```python
from build123d import *

# Parameters (mm, degrees)
F0_R     = 2.55
F1_DEPTH = 6.1
F3_DEPTH = 2.5
F6_DEPTH = 1.2


with BuildPart() as f1:
    # F0 (on Top) → F1 (new body)
    with BuildSketch(Plane.XY):
        with BuildLine():
            ThreePointArc((-22.8091472875, 20.7166310371), (-24.4512119604, 22.7321355607), (-25.1048969271, 25.2483491523))
            ThreePointArc((-25.1048969271, 25.2483491523), (-34.1357153903, 30.6750208196), (-35.5153225806, 20.2298721131))
            ThreePointArc((-35.5153225806, 20.2298721131), (-33.9539864651, 18.15120321), (-33.4, 15.6111768576))
            Line((-33.4, 15.6111768576), (-33.4, -15.6111768576))
            ThreePointArc((-33.4, -15.6111768576), (-33.9539864651, -18.15120321), (-35.5153225806, -20.2298721131))
            ThreePointArc((-35.5153225806, -20.2298721131), (-34.1357149704, -30.6750210221), (-25.1048968903, -25.2483482207))
            ThreePointArc((-25.1048968903, -25.2483482207), (-24.4512125214, -22.7321357825), (-22.8091487233, -20.7166321802))
            Line((-22.8091487233, -20.7166321802), (-16.801235426, -15.9332617206))
            ThreePointArc((-16.801235426, -15.9332617206), (-16.4823258273, -13.1228708816), (-19.2927166663, -12.8039612829))
            Line((-19.2927166663, -12.8039612829), (-25.3006299635, -17.5873317424))
            ThreePointArc((-25.3006299635, -17.5873317424), (-27.9708920533, -17.8865901621), (-29.4, -15.6111768576))
            Line((-29.4, -15.6111768576), (-29.4, 15.6111768576))
            ThreePointArc((-29.4, 15.6111768576), (-27.9708912267, 17.8865905605), (-25.3006285278, 17.5873305993))
            Line((-25.3006285278, 17.5873305993), (-8.5908527125, 4.2833689629))
            ThreePointArc((-8.5908527125, 4.2833689629), (-6.5260006587, 0), (-8.5908527125, -4.2833689629))
            Line((-8.5908527125, -4.2833689629), (-14.5987660097, -9.0667394225))
            ThreePointArc((-14.5987660097, -9.0667394225), (-14.9176756084, -11.8771302615), (-12.1072847694, -12.1960398602))
            Line((-12.1072847694, -12.1960398602), (-6.0993714722, -7.4126694007))
            ThreePointArc((-6.0993714722, -7.4126694007), (-3.7671833568, -6.2639599209), (-1.1684785693, -6.1906912242))
            ThreePointArc((-1.1684785693, -6.1906912242), (6.3, 0), (-1.1684785693, 6.1906912242))
            ThreePointArc((-1.1684785693, 6.1906912242), (-3.7671833568, 6.2639599209), (-6.0993714722, 7.4126694007))
            Line((-6.0993714722, 7.4126694007), (-22.8091472875, 20.7166310371))
        make_face()
        with Locations((-31.4, -25)):
            Circle(F0_R, mode=Mode.SUBTRACT)
        with Locations((-31.4, 25)):
            Circle(F0_R, mode=Mode.SUBTRACT)
        Circle(F0_R, mode=Mode.SUBTRACT)
    extrude(amount=F1_DEPTH)

    # F2 (on face) → F3 (cut)
    with BuildSketch(Plane.XY.offset(6.1)):
        Polygon((-27.35, 22.6617314098), (-27.35, 27.3382685902), (-31.4, 29.6765371804), (-35.45, 27.3382685902), (-35.45, 22.6617314098), (-31.4, 20.3234628196), align=None)
        Polygon((-27.35, -27.3382685902), (-27.35, -22.6617314098), (-31.4, -20.3234628196), (-35.45, -22.6617314098), (-35.45, -27.3382685902), (-31.4, -29.6765371804), align=None)
        Polygon((-4.05, 2.3382685902), (-4.05, -2.3382685902), (0, -4.6765371804), (4.05, -2.3382685902), (4.05, 2.3382685902), (0, 4.6765371804), align=None)
    extrude(amount=-F3_DEPTH, mode=Mode.SUBTRACT)

    # F5 (on mid) → F6 (cut, symmetric)
    with BuildSketch(Plane.XY.offset(3.05)):
        with BuildLine():
            Line((-19.2927166663, -12.8039612829), (-21.5397744668, -14.5930200413))
            ThreePointArc((-21.5397744668, -14.5930200413), (-20.7851139292, -16.5486575869), (-19.0482932266, -17.722320479))
            Line((-19.0482932266, -17.722320479), (-16.801235426, -15.9332617206))
            ThreePointArc((-16.801235426, -15.9332617206), (-19.611626265, -15.6143521218), (-19.2927166663, -12.8039612829))
        make_face()
        with BuildLine():
            ThreePointArc((-14.5987660097, -9.0667394225), (-11.7883751707, -9.3856490213), (-12.1072847694, -12.1960398602))
            Line((-12.1072847694, -12.1960398602), (-9.8602269689, -10.4069811018))
            ThreePointArc((-9.8602269689, -10.4069811018), (-10.6148875066, -8.4513435562), (-12.3517082091, -7.2776806641))
            Line((-12.3517082091, -7.2776806641), (-14.5987660097, -9.0667394225))
        make_face()
    extrude(amount=F6_DEPTH, both=True, mode=Mode.SUBTRACT)


solid = f1.part
```
Can you work these out from the model? Positions are in its coordinate system, mm. A direction names the side the tool comes from. Coordinates: 2 decimals unless noted, no trailing zeros. Order: outer loops, then holes, each group sorted by start corner. A loop starts at its lowest first (then second) coordinate and runs counter-clockwise, first axis right, second up.
1. If we section it at C-C (y = -19): Please give me the cut outline in (x, z).
2. Thinking about a two-plate mould opening in X: for faces 6 (the face through (-33.969, 18.185, 3.007)), 7 (the face through (-24.468, -22.765, 3.007)), 8 (the face through (-30.03, 27.15, 1.77)), which applies, +X half, -X half, draft (parallel to the pull), parting line (faces both ways), or undercut?
3. I'm going to push flat-ended pins straight in: pin 1 (3 mm diameter, centred on y = 0, z = 4.5, fed in from -X); pin 2 (3 mm diameter, centred on x = -4, z = 4.5, fed in from -Y); pin 3 (1 mm diameter, centred on y = -18, z = 1.5, fed in from -X). Where does each tip first touch, or does it pass through?
4. If we section it at A-A (y = 0): Please give me the cut outline in (x, z).
5. If we section it at B-B (z = 2.75): Please give me the cut outline in (x, y).
6. I need wall thicknesses on line 1 (Y direction, x = -31.4, z = 1.9); line 2 (Y direction, x = 0, z = 1.95); line 3 (X direction, y = -3.5, z = 5). Which ranges of each line are inside material? Lowest first, please.
7. For faces 1 (the face through (-17.063, 11.028, 3.007)), 2 (the face through (-2, -2, 3.6)), 3 (the face through (-3.803, -6.273, 3.007)), 4 (the face through (-20.8, -16.53, 3.03)), 5 (the face through (-33.94, -18.12, 3.01)), which set-ups out of +Z, -Z, +X, -X, +Y, -Y let a thin tool reach every point of the face, with its end or its side?
Entries:
1. outline: (-34.43, 0) - (-20.65, 0) - (-20.65, 6.1) - (-34.43, 6.1) - close
2. face 6: -X half
2. face 7: +X half
2. face 8: undercut
3. pin 1: stops at x = -33.4
3. pin 2: stops at y = -6.99
3. pin 3: stops at x = -34.13
4. outline: (-33.4, 0) - (-29.4, 0) - (-29.4, 6.1) - (-33.4, 6.1) - close; (-6.53, 0) - (-2.55, 0) - (-2.55, 3.6) - (-4.05, 3.6) - (-4.05, 6.1) - (-6.53, 6.1) - close; (2.55, 0) - (6.3, 0) - (6.3, 6.1) - (4.05, 6.1) - (4.05, 3.6) - (2.55, 3.6) - close
5. outline: (-35.52, -20.23) arc R6.3 ccw (long way) to (-25.1, -25.25) arc R6.1 cw to (-22.81, -20.72) - (-19.05, -17.72) arc R3.5 cw to (-21.54, -14.59) - (-25.3, -17.59) arc R2.53 cw to (-29.4, -15.61) - (-29.4, 15.61) arc R2.53 cw to (-25.3, 17.59) - (-8.59, 4.28) arc R5.48 cw to (-8.59, -4.28) - (-12.35, -7.28) arc R3.5 cw to (-9.86, -10.41) - (-6.1, -7.41) arc R6.1 cw to (-1.17, -6.19) arc R6.3 ccw (long way) to (-1.17, 6.19) arc R6.1 cw to (-6.1, 7.41) - (-22.81, 20.72) arc R6.1 cw to (-25.1, 25.25) arc R6.3 ccw (long way) to (-35.52, 20.23) arc R6.1 cw to (-33.4, 15.61) - (-33.4, -15.61) arc R6.1 cw to start; circle Ø4 at (-18.05, -14.37); circle Ø4 at (-13.35, -10.63); hole circle Ø5.1 at (-31.4, -25); hole circle Ø5.1 at (-31.4, 25); hole circle Ø5.1 at (0, 0)
6. line 1: y = -31.3 to -27.55, -22.45 to 22.45, 27.55 to 31.3
6. line 2: y = -6.3 to -2.55, 2.55 to 6.3
6. line 3: x = -33.4 to -29.4, -7.79 to -2.04, 2.04 to 5.24
7. face 1: +Z, -Z
7. face 2: +Z
7. face 3: +Z, -Z, -Y
7. face 4: none
7. face 5: +Z, -Z, -X
